```python
from build123d import *

# Parameters (mm, degrees)
ESQUISSE1_W             = 54
ESQUISSE1_H             = 18
ESQUISSE1_R             = 3
BOSS_EXTRU_1_DEPTH      = 57
ENL_V_MAT_EXTRU_1_DEPTH = 57


with BuildPart() as part:
    # Esquisse1 → Boss.-Extru.1 (new body)
    with BuildSketch(Plane.XY):
        with Locations((0, -9)):
            Rectangle(ESQUISSE1_W, ESQUISSE1_H)
        with Locations(Location((-20, -8, 0), (0, 0, 180))):
            Circle(ESQUISSE1_R, mode=Mode.SUBTRACT)
        with Locations(Location((20, -8, 0), (0, 0, 180))):
            Circle(ESQUISSE1_R, mode=Mode.SUBTRACT)
    extrude(amount=BOSS_EXTRU_1_DEPTH)

    # Esquisse3 → Enlèv. mat.-Extru.1 (cut)
    with BuildSketch(Plane.ZY.offset(27)):
        with BuildLine():
            Line((52, 0), (5, 0))
            Line((5, 0), (5, -11))
            ThreePointArc((5, -11), (5.585786438, -12.414213562), (7, -13))
            Line((7, -13), (50, -13))
            ThreePointArc((50, -13), (51.414213562, -12.414213562), (52, -11))
            Line((52, -11), (52, 0))
        make_face()
    extrude(amount=-ENL_V_MAT_EXTRU_1_DEPTH, mode=Mode.SUBTRACT)


solid = part.part
```
Geometry check sheet. Reference: the model listing, model coordinates, mm. A direction names the side the tool comes from. Coordinates: 2 decimals unless noted, no trailing zeros. Loops run counter-clockwise (first coordinate to the right, second up) from the corner with the lowest first, then second, coordinate; pieces in that order, holes last. Notation, with made-up numbers: (-4, 84) -> (43, 84) arc R21 ccw to (43, 102) -> close; hole circle Ø6 at (35, 51). An arc over 180 degrees is marked (long way). Put each result on its own line as item: value.
1) Release check for a two-part mould opening along Y. For faces 1 (the flat face through (0, 0, 2)), 2 (the flat face through (-27, -15, 28)), 3 (the cylindrical face through (-17, -8, 54)) record: released by +Y, released by -Y, zero draft, split by the parting line, or undercut.
Result set:
face 1: released by +Y
face 2: zero draft
face 3: undercut
2) Cross-section at A-A on y = -8. Record the boundary of the cut face in (x, z).
Result set:
outline: (-27, 0) -> (-23, 0) -> (-23, 5) -> (-27, 5) -> close; (-27, 52) -> (-23, 52) -> (-23, 57) -> (-27, 57) -> close; (-17, 0) -> (17, 0) -> (17, 5) -> (-17, 5) -> close; (-17, 52) -> (17, 52) -> (17, 57) -> (-17, 57) -> close; (23, 0) -> (27, 0) -> (27, 5) -> (23, 5) -> close; (23, 52) -> (27, 52) -> (27, 57) -> (23, 57) -> close
3) Tool access check on faces 4 (the flat face through (0, -13, 28)), 5 (the flat face through (0, -18, 28)). Record the directions out of +Z, -Z, +X, -X, +Y, -Y that give a thin tool (end or side, any length) a straight path to the whole face; none if there is none.
Result set:
face 4: +X, -X, +Y
face 5: +Z, -Z, +X, -X, -Y
4) Cross-section at B-B on x = 15. Record the boundary of the cut face in (y, z).
Result set:
outline: (-18, 0) -> (0, 0) -> (0, 5) -> (-11, 5) arc R2 cw to (-13, 7) -> (-13, 50) arc R2 cw to (-11, 52) -> (0, 52) -> (0, 57) -> (-18, 57) -> close
5) Cross-section at C-C on z = 30. Record the boundary of the cut face in (x, y).
Result set:
outline: (-27, -18) -> (27, -18) -> (27, -13) -> (-27, -13) -> close
6) Thickness scan on line 1 (X direction, y = -8, z = 1.95); line 2 (Z direction, x = 2.5, y = -9.5); line 3 (Y direction, x = 20, z = 3.65). Record the ranges inside material, lowest first.
Result set:
line 1: x = -27 to -23, -17 to 17, 23 to 27
line 2: z = 0 to 5, 52 to 57
line 3: y = -18 to -11, -5 to 0
